Input: part model. Units: mm. Frame: model coordinates. A direction names the side the tool comes from. Give positions to 0.01 mm unless a question says otherwise; leave off trailing zeros. Write each loop counter-clockwise with the first axis right and the second up, starting at its lowest first coordinate (ties: lowest second). Pieces come first, ordered by that corner, then holes.
```python
from build123d import *

# Parameters (mm, degrees)
BOSS_EXTRUDE1_DEPTH = 60
BOSS_EXTRUDE2_DEPTH = 10


with BuildPart() as part:
    # Sketch1 → Boss-Extrude1 (new body)
    with BuildSketch(Plane(origin=(0, 0, 0), x_dir=(1, 0, 0), z_dir=(0, 1, 0))):
        Polygon((72.260273973, 79.863013699), (-107.739726027, 79.863013699), (-107.739726027, 29.863013699), (-70.739726027, 29.863013699), (-70.739726027, -80.136986301), (-117.739726027, -80.136986301), (-117.739726027, -150.136986301), (82.260273973, -150.136986301), (82.260273973, -80.136986301), (35.260273973, -80.136986301), (35.260273973, 29.863013699), (72.260273973, 29.863013699), align=None)
        Polygon((69.260273973, 76.863013699), (-104.739726027, 76.863013699), (-104.739726027, 32.863013699), (-67.739726027, 32.863013699), (-67.739726027, -83.136986301), (-114.739726027, -83.136986301), (-114.739726027, -147.136986301), (79.260273973, -147.136986301), (79.260273973, -83.136986301), (32.260273973, -83.136986301), (32.260273973, 32.863013699), (69.260273973, 32.863013699), align=None, mode=Mode.SUBTRACT)
    extrude(amount=BOSS_EXTRUDE1_DEPTH)

    # Sketch2 → Boss-Extrude2 (add)
    with BuildSketch(Plane(origin=(0, 0, 0), x_dir=(1, 0, 0), z_dir=(0, 1, 0))):
        Polygon((72.260273973, 29.863013699), (72.260273973, 79.863013699), (-107.739726027, 79.863013699), (-107.739726027, 29.863013699), (-70.739726027, 29.863013699), (-70.739726027, -80.136986301), (-117.739726027, -80.136986301), (-117.739726027, -150.136986301), (82.260273973, -150.136986301), (82.260273973, -80.136986301), (35.260273973, -80.136986301), (35.260273973, 29.863013699), align=None)
    extrude(amount=-BOSS_EXTRUDE2_DEPTH)


solid = part.part
```
Q1. Section A-A, the plane x = 38.5. Return the cut outline in (y, z).
Q2. Section D-D, the plane x = -40.5. Return the cut outline in (y, z).
Q3. Pin query (flat end, axial travel): pin 1 (2 mm diameter, centred on x = -36, z = -1, fed in from +Y); pin 2 (10 mm diameter, centred on y = 45.5, z = 39.5, fed in from -X); pin 3 (22 mm diameter, centred on y = 22.5, z = -57.5, fed in from -X). Return the tip coordinate at first contact, or that it passes through.
Q4. Section C-C, the plane z = 23.5. Return the cut outline in (x, y).
Q5. Section B-B, the plane y = 45. Return the cut outline in (x, z).
Q6. Access query for faces 5 (the flat face through (-70.74, 25, 24)), 6 (the flat face through (-86, 30, -32.863)), 7 (the flat face through (59, 25, 80.137)). Directions: +Z, -Z, +X, -X, +Y, -Y. A direction counts if a zero-diameter tool reaches every point of the face in a straight line with its end or side. Return the directions, or none.
Q7. Material intervals for line 1 along Z through (x, y) = (33, 27.5); line 2 along Z through (x, y) = (-74, 17); line 3 along Z through (x, y) = (-13, 39.5), sorted ascending.
Q8. Mould query, pull axis X, two halves, no side actions, for faces 1 (the flat face through (-107.74, 25, -55)), 2 (the flat face through (34, 60, 1)), 3 (the flat face through (51, 30, -32.863)), 4 (the flat face through (35.26, 25, 26)). Classes: +X half, -X half, draft (parallel to the pull), parting line (faces both ways), or undercut.
Solutions:
1. outline: (-10, -79.86) - (60, -79.86) - (60, -76.86) - (0, -76.86) - (0, -32.86) - (60, -32.86) - (60, -29.86) - (-10, -29.86) - close; (-10, 80.14) - (60, 80.14) - (60, 83.14) - (0, 83.14) - (0, 147.14) - (60, 147.14) - (60, 150.14) - (-10, 150.14) - close
2. outline: (-10, -79.86) - (60, -79.86) - (60, -76.86) - (0, -76.86) - (0, 147.14) - (60, 147.14) - (60, 150.14) - (-10, 150.14) - close
3. pin 1: stops at y = 0
3. pin 2: stops at x = -70.74
3. pin 3: stops at x = -107.74
4. outline: (-70.74, -10) - (35.26, -10) - (35.26, 60) - (32.26, 60) - (32.26, 0) - (-67.74, 0) - (-67.74, 60) - (-70.74, 60) - close
5. outline: (-117.74, 80.14) - (-70.74, 80.14) - (-70.74, -29.86) - (-107.74, -29.86) - (-107.74, -79.86) - (72.26, -79.86) - (72.26, -29.86) - (35.26, -29.86) - (35.26, 80.14) - (82.26, 80.14) - (82.26, 150.14) - (-117.74, 150.14) - close; hole (-114.74, 83.14) - (-67.74, 83.14) - (-67.74, -32.86) - (-104.74, -32.86) - (-104.74, -76.86) - (69.26, -76.86) - (69.26, -32.86) - (32.26, -32.86) - (32.26, 83.14) - (79.26, 83.14) - (79.26, 147.14) - (-114.74, 147.14) - close
6. face 5: -X, +Y, -Y
6. face 6: +Y
6. face 7: +X, +Y, -Y
7. line 1: z = -79.86 to -76.86, -32.86 to 83.14, 147.14 to 150.14
7. line 2: z = -79.86 to -76.86, -32.86 to -29.86, 80.14 to 83.14, 147.14 to 150.14
7. line 3: z = -79.86 to -76.86, 147.14 to 150.14
8. face 1: -X half
8. face 2: draft
8. face 3: undercut
8. face 4: +X half
